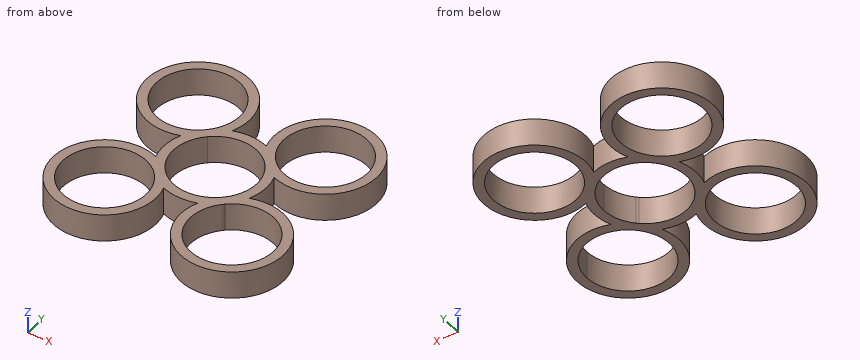
```python
from build123d import *

# Parameters (mm, degrees)
F5_DEPTH = 7.239
F1_R     = 13.5382
F1_R_2   = 10.9982
F6_DEPTH = 7.239
F2_R     = 13.5382
F2_R_2   = 10.9982
F7_DEPTH = 7.239
F3_R     = 13.5382
F3_R_2   = 10.9982
F8_DEPTH = 7.239
F4_R     = 13.5382
F4_R_2   = 10.9982
F9_DEPTH = 7.239


with BuildPart() as f5:
    # F0 (on Top) → F5 (new body)
    with BuildSketch(Plane.XY):
        with BuildLine():
            ThreePointArc((7.98923, 7.561236), (10.219629, 4.069307), (11.000003, 0))
            ThreePointArc((11.000003, 0), (10.103804, -4.348934), (7.561236, -7.98923))
            Line((7.561236, -7.98923), (9.307193, -9.834015))
            ThreePointArc((9.307193, -9.834015), (9.478103, -9.661638), (9.653725, -9.494066))
            ThreePointArc((9.653725, -9.494066), (13.539381, -0.129832), (9.834015, 9.307193))
            Line((9.834015, 9.307193), (7.98923, 7.561236))
        make_face()
        with BuildLine():
            ThreePointArc((-7.561236, 7.98923), (0.302638, 10.995839), (7.98923, 7.561236))
            Line((7.98923, 7.561236), (9.834015, 9.307193))
            ThreePointArc((9.834015, 9.307193), (0.372519, 13.534878), (-9.307193, 9.834015))
            Line((-9.307193, 9.834015), (-7.561236, 7.98923))
        make_face()
        with BuildLine():
            Line((9.307193, -9.834015), (7.561236, -7.98923))
            ThreePointArc((7.561236, -7.98923), (-0.302638, -10.995839), (-7.98923, -7.561236))
            Line((-7.98923, -7.561236), (-9.834015, -9.307193))
            ThreePointArc((-9.834015, -9.307193), (-0.372519, -13.534878), (9.307193, -9.834015))
        make_face()
        with BuildLine():
            ThreePointArc((-7.98923, -7.561236), (-10.995839, 0.302638), (-7.561236, 7.98923))
            Line((-7.561236, 7.98923), (-9.307193, 9.834015))
            ThreePointArc((-9.307193, 9.834015), (-13.534878, 0.372519), (-9.834015, -9.307193))
            Line((-9.834015, -9.307193), (-7.98923, -7.561236))
        make_face()
    extrude(amount=F5_DEPTH)

    # F1 (on Top) → F6 (join)
    with BuildSketch(Plane.XY):
        with Locations((16.860046, -17.814388)):
            Circle(F1_R)
        with Locations((16.860046, -17.814388)):
            Circle(F1_R_2, mode=Mode.SUBTRACT)
    extrude(amount=F6_DEPTH)

    # F2 (on Top) → F7 (join)
    with BuildSketch(Plane.XY):
        with Locations((-17.821935, -16.867189)):
            Circle(F2_R)
        with Locations((-17.821935, -16.867189)):
            Circle(F2_R_2, mode=Mode.SUBTRACT)
    extrude(amount=F7_DEPTH)

    # F3 (on Top) → F8 (join)
    with BuildSketch(Plane.XY):
        with Locations((-16.867189, 17.821935)):
            Circle(F3_R)
        with Locations((-16.867189, 17.821935)):
            Circle(F3_R_2, mode=Mode.SUBTRACT)
    extrude(amount=F8_DEPTH)

    # F4 (on Top) → F9 (join)
    with BuildSketch(Plane.XY):
        with Locations((17.821935, 16.867189)):
            Circle(F4_R)
        with Locations((17.821935, 16.867189)):
            Circle(F4_R_2, mode=Mode.SUBTRACT)
    extrude(amount=F9_DEPTH)


solid = f5.part
```
Input: part model. Units: mm. Frame: model coordinates. Give positions to 0.01 mm unless a question says otherwise; leave off trailing zeros. Order: outer loops, then holes, each group sorted by start corner. A loop starts at its lowest first (then second) coordinate and runs counter-clockwise, first axis right, second up. Notation, with made-up numbers: (47.5, 20) -> (76.5, 20) arc R21 cw to (76.5, 33) -> close; hole circle Ø1 at (59.5, -38.75). An arc over 180 degrees is marked (long way). Write each question's results on one line, items separated by ' | '. Start each with the question number.
Item 1: Cut plane B-B on y = 19. Return the cut outline in (x, z).
Item 2: Cut plane A-A on x = 15. Return the cut outline in (y, z).
Item 3: Line query: line 1 (Y direction, x = 0, z = 5.25); line 2 (Y direction, x = -15.5, z = 3.5); line 3 (X direction, y = -26, z = 4.25). Output: solid intervals per line, ascending.
Item 4: Cut plane C-C on z = 3.25. Give the number of separate pieces and of enclosed holes in the cut face, then the cut area to 3 significant figures.
Item 5: Contact query for flat-ended pins moving along their axis: P1, Ø1, axis at y = -15, z = 1, coming from the +X side; P2, Ø4, axis at x = 12, z = 4.5, coming from the +Y side. Output: stop coordinate, or through.
Established:
1) outline: (-30.35, 0) -> (-27.8, 0) -> (-27.8, 7.24) -> (-30.35, 7.24) -> close; (-5.93, 0) -> (-3.38, 0) -> (-3.38, 7.24) -> (-5.93, 7.24) -> close; (4.45, 0) -> (7.03, 0) -> (7.03, 7.24) -> (4.45, 7.24) -> close; (28.61, 0) -> (31.19, 0) -> (31.19, 7.24) -> (28.61, 7.24) -> close
2) outline: (-31.22, 0) -> (-28.65, 0) -> (-28.65, 7.24) -> (-31.22, 7.24) -> close; (-6.97, 0) -> (-4.4, 0) -> (-4.4, 7.24) -> (-6.97, 7.24) -> close; (3.63, 0) -> (6.24, 0) -> (6.24, 7.24) -> (3.63, 7.24) -> close; (27.5, 0) -> (30.11, 0) -> (30.11, 7.24) -> (27.5, 7.24) -> close
3) line 1: -13.54 to -11, 11 to 13.54 | line 2: -30.2 to -27.62, -6.12 to -3.53, 4.35 to 6.91, 28.73 to 31.29 | line 3: -27.82 to -23.95, -11.69 to -7.83, 6.08 to 9.51, 24.21 to 27.64
4) separate pieces: 1 | enclosed holes: 5 | area: 901 mm^2
5) P1: x = 30.2 | P2: y = 29.85
